CAD build for the part. Positions are in the model's coordinates, mm. Face numbers are marked on the shaded views. A direction names the side the tool comes from. Coordinates: 2 decimals unless noted, no trailing zeros. Loops run counter-clockwise (first coordinate to the right, second up) from the corner with the lowest first, then second, coordinate; pieces in that order, holes last. Notation, with made-up numbers: (-2, -19) -> (39, -19) arc R37 cw to (39, 18) -> close; hole circle Ø5 at (52, 68). An arc over 180 degrees is marked (long way). Return JSON: item names as keys, results as strings. Group by question number.
(1) Saw through at C-C on y = -4.75. Write the cut outline in (x, z), then the cut area to 3 significant figures.
(2) Saw through at B-B on x = 24.5. Write the cut outline in (y, z), then the cut area to 3 significant figures.
(3) Saw through at A-A on z = 12. Write the cut outline in (x, y).
(4) Tool access for the marked faces 4, 5, 6, 7 and 8: list every direction of +Z, -Z, +X, -X, +Y, -Y with a clear straight run to the whole face (end or side of a thin tool).
(5) Flat gauge pins, fed straight in: pin 1 Ø6 at (x, y) = (13, 3.5) entering from -Z; pin 2 Ø1.7 at (x, z) = (15.5, 0) entering from -Y; pin 3 Ø1.4 at (x, z) = (-2, 0) entering from -Y. Where does each tip first touch, or does it go through?
(6) Saw through at D-D on z = 0. Write the cut outline in (x, y).
(7) Probe L1, parallel to X at y = -7, z = 0; L2, parallel to X at y = -4.5, z = 0; L3, parallel to X at y = 1.75, z = -8. List the from-to ranges inside material, lowest first.
(8) Mould opens along X. For the marked faces 1, 2 and 3 say: pulls with the +X half, pulls with the -X half, needs draft (parallel to the pull), parting line crosses it, or undercut.
```python
from build123d import *

# Parameters (mm, degrees)
SKETCH1_W           = 13.8
SKETCH1_H           = 10.5
BOSS_EXTRUDE1_DEPTH = 22
BOSS_EXTRUDE2_DEPTH = 5
BOSS_EXTRUDE3_DEPTH = 5
SKETCH4_R           = 1.4
CUT_EXTRUDE1_DEPTH  = 8
SKETCH5_W           = 22
SKETCH5_H           = 10.1
CUT_EXTRUDE2_DEPTH  = 37.390245946
FILLET2_R           = 1
FILLET3_R           = 4


with BuildPart() as part:
    # Sketch1 → Boss-Extrude1 (new body)
    with BuildSketch(Plane(origin=(0, 0, 0), x_dir=(0, 0, -1), z_dir=(1, 0, 0))):
        Polygon((6.9, 5.25), (17, 5.25), (17, 7.25), (-17, 7.25), (-17, 5.25), (-6.9, 5.25), align=None)
        Rectangle(SKETCH1_W, SKETCH1_H)
    extrude(amount=BOSS_EXTRUDE1_DEPTH)

    # Sketch2 → Boss-Extrude2 (add)
    with BuildSketch(Plane(origin=(22, 0, 0), x_dir=(0, 0, -1), z_dir=(1, 0, 0))):
        Polygon((-6.9, 5.25), (-17, 5.25), (-17, -10.25), (17, -10.25), (17, 5.25), (6.9, 5.25), (6.9, -5.25), (-6.9, -5.25), align=None)
        Polygon((-17, 7.25), (-17, 5.25), (-6.9, 5.25), (-6.9, -5.25), (6.9, -5.25), (6.9, 5.25), (17, 5.25), (17, 7.25), align=None)
    extrude(amount=BOSS_EXTRUDE2_DEPTH)

    # Sketch3 → Boss-Extrude3 (add)
    with BuildSketch(Plane.ZY):
        Polygon((17, -10.25), (17, 5.25), (6.9, 5.25), (6.9, -5.25), (-6.9, -5.25), (-6.9, 5.25), (-17, 5.25), (-17, -10.25), align=None)
        Polygon((6.9, -5.25), (6.9, 5.25), (17, 5.25), (17, 7.25), (-17, 7.25), (-17, 5.25), (-6.9, 5.25), (-6.9, -5.25), align=None)
    extrude(amount=BOSS_EXTRUDE3_DEPTH)

    # Sketch4 → Cut-Extrude1 (cut)
    with BuildSketch(Plane.XZ.offset(10.25)):
        with Locations(Location((-2.5, 0, 0), (0, 0, 270))):
            Circle(SKETCH4_R)
        with Locations(Location((24.5, 0, 0), (0, 0, 270))):
            Circle(SKETCH4_R)
    extrude(amount=-CUT_EXTRUDE1_DEPTH, mode=Mode.SUBTRACT)

    # Sketch5 → Cut-Extrude2 (cut, through all)
    with BuildSketch(Plane(origin=(0, 7.25, 0), x_dir=(1, 0, 0), z_dir=(0, 1, 0))):
        with Locations((11, -11.95)):
            Rectangle(SKETCH5_W, SKETCH5_H)
        with Locations((11, 11.95)):
            Rectangle(SKETCH5_W, SKETCH5_H)
    extrude(amount=-CUT_EXTRUDE2_DEPTH, mode=Mode.SUBTRACT)

    # Fillet2
    fillet2_edges = [part.edges().sort_by_distance(p)[0] for p in [
        (24.5, 7.25, 17),
        (24.5, 7.25, -17),
        (22, -1.5, -17),
        (27, -1.5, -17),
        (22, -1.5, 17),
        (27, 7.25, 0),
        (27, -1.5, 17),
        (-5, -1.5, 17),
        (0, -1.5, -17),
        (-5, 7.25, 0),
        (-5, -1.5, -17),
        (0, -1.5, 17),
        (-2.5, 7.25, 17),
        (-2.5, 7.25, -17),
        (22, 7.25, 11.95),
        (11, 7.25, 6.9),
        (0, 7.25, 11.95),
        (11, 7.25, -6.9),
        (22, 7.25, -11.95),
        (0, 7.25, -11.95),
    ]]
    fillet(fillet2_edges, radius=FILLET2_R)

    # Fillet3
    fillet3_edges = [part.edges().sort_by_distance(p)[0] for p in [
        (11, -5.25, -6.9),
        (11, -5.25, 6.9),
    ]]
    fillet(fillet3_edges, radius=FILLET3_R)


solid = part.part
```
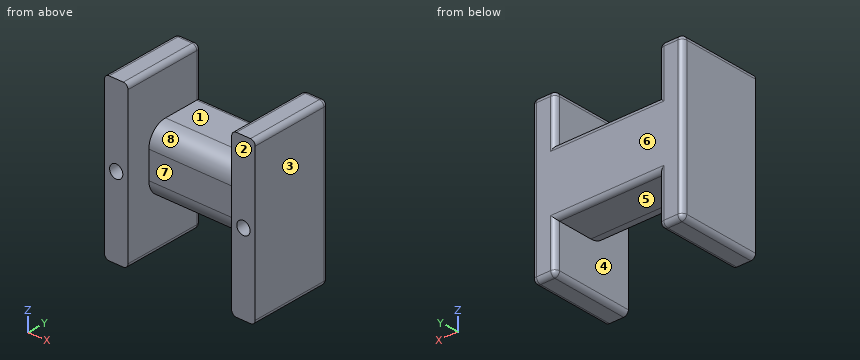
Geometry results:
{
 "1": {"outline": "(-5, -16) arc R1 ccw to (-4, -17) -> (-1, -17) arc R1 ccw to (0, -16) -> (0, -4.84) -> (22, -4.84) -> (22, -16) arc R1 ccw to (23, -17) -> (26, -17) arc R1 ccw to (27, -16) -> (27, 16) arc R1 ccw to (26, 17) -> (23, 17) arc R1 ccw to (22, 16) -> (22, 4.84) -> (0, 4.84) -> (0, 16) arc R1 ccw to (-1, 17) -> (-4, 17) arc R1 ccw to (-5, 16) -> close; hole circle Ø2.8 at (-2.5, 0); hole circle Ø2.8 at (24.5, 0)", "area": "539 mm²"},
 "2": {"outline": "(-10.25, -17) -> (6.25, -17) arc R1 ccw to (7.25, -16) -> (7.25, 16) arc R1 ccw to (6.25, 17) -> (-10.25, 17) -> (-10.25, 1.4) -> (-2.25, 1.4) -> (-2.25, -1.4) -> (-10.25, -1.4) -> close", "area": "572 mm²"},
 "3": {"outline": "(-5, -10.25) -> (0, -10.25) -> (0, 6.25) arc R1 ccw to (-1, 7.25) -> (-4, 7.25) arc R1 ccw to (-5, 6.25) -> close; (22, -10.25) -> (27, -10.25) -> (27, 6.25) arc R1 ccw to (26, 7.25) -> (23, 7.25) arc R1 ccw to (22, 6.25) -> close"},
 "4": {"face 4": "-Y", "face 5": "-Z, +Y, -Y", "face 6": "+Z, -Z, +X, -X, +Y", "face 7": "+Z, -Z, -Y", "face 8": "+Z, -Y"},
 "5": {"pin 1": "z = -6.9", "pin 2": "y = -5.25", "pin 3": "y = -2.25"},
 "6": {"outline": "(-5, -10.25) -> (-3.9, -10.25) -> (-3.9, -2.25) -> (-1.1, -2.25) -> (-1.1, -10.25) -> (0, -10.25) -> (0, -5.25) -> (22, -5.25) -> (22, -10.25) -> (23.1, -10.25) -> (23.1, -2.25) -> (25.9, -2.25) -> (25.9, -10.25) -> (27, -10.25) -> (27, 6.25) arc R1 ccw to (26, 7.25) -> (-4, 7.25) arc R1 ccw to (-5, 6.25) -> close"},
 "7": {"L1": "-5 to -3.9, -1.1 to 0, 22 to 23.1, 25.9 to 27", "L2": "-5 to -3.9, -1.1 to 23.1, 25.9 to 27", "L3": "-5 to 0, 22 to 27"},
 "8": {"face 1": "undercut", "face 2": "needs draft", "face 3": "pulls with the +X half"}
}
